Design review of the part shown in the three views and the two pictorial views. Dimensions are in mm from the part's minimum x, y and z. A direction names the side the tool comes from. Give positions to 0.01 mm unless a question says otherwise; leave off trailing zeros. Write each loop counter-clockwise with the first axis right and the second up, starting at its lowest first coordinate (ties: lowest second). Pieces come first, ordered by that corner, then holes. Notation, with made-up numbers: M 68,-32 L 90,-32 A17 ccw 90,-10 Z; hole C -17,67 d2. An arc over 180 degrees is marked long. Write item = value, one per line.
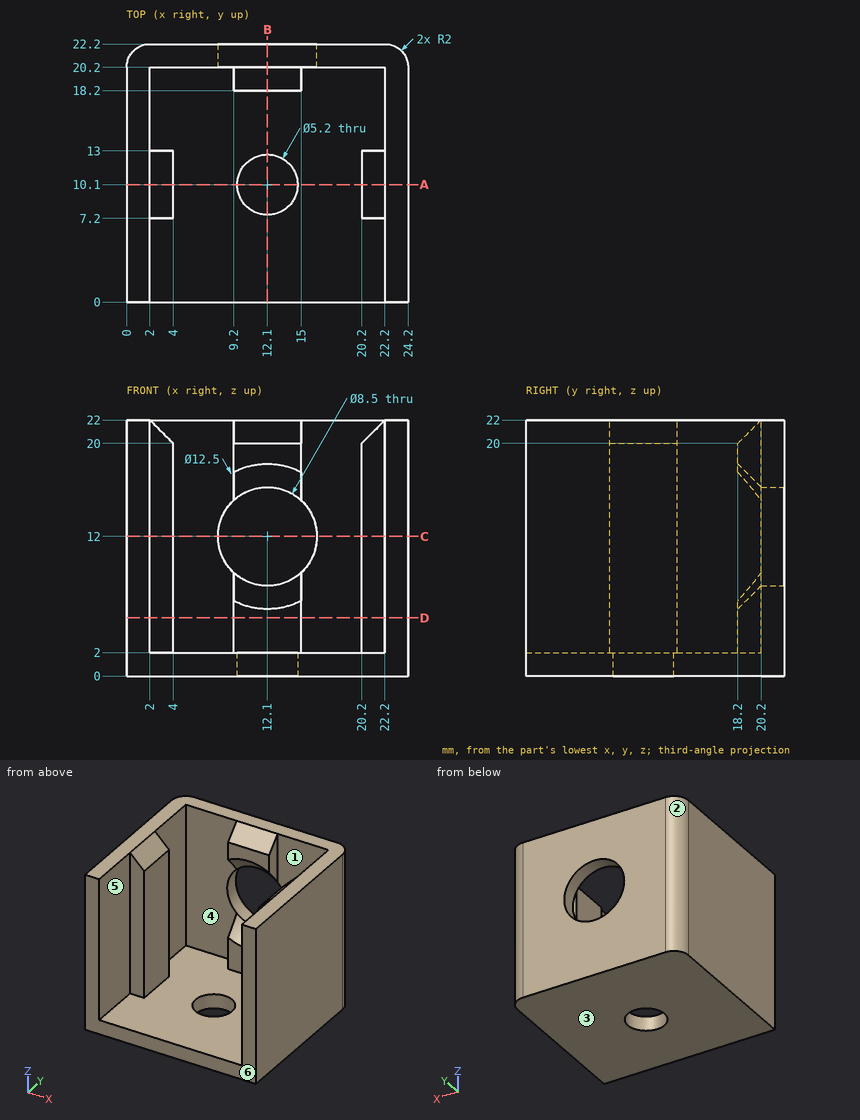
1. We need section D-D, the plane z = 5. Write out the cut boundary in (x, y), then the cut area to 3 significant figures.
Responses:
outline = M 0,0 L 2,0 L 2,7.2 L 4,7.2 L 4,13 L 2,13 L 2,20.2 L 9.2,20.2 L 9.2,18.2 L 15,18.2 L 15,20.2 L 22.2,20.2 L 22.2,13 L 20.2,13 L 20.2,7.2 L 22.2,7.2 L 22.2,0 L 24.2,0 L 24.2,20.2 A2 ccw 22.2,22.2 L 2,22.2 A2 ccw 0,20.2 Z
area = 162 mm2
2. Machinability: for the marked faces 4, 5 and 6, which of the approach directions +Z, -Z, +X, -X, +Y, -Y give a long, thin tool a straight path to every point of the face, cutting with its end or side? Answer none if there is none.
Responses:
face_4 = +Z
face_5 = +Z, -Y
face_6 = +Z, -Z, +X, -X, -Y
3. We need section C-C, the plane z = 12. Write out the cut boundary in (x, y), then the cut area to 3 significant figures.
Responses:
outline = M 0,0 L 2,0 L 2,7.2 L 4,7.2 L 4,13 L 2,13 L 2,20.2 L 7.85,20.2 L 7.85,22.2 L 2,22.2 A2 ccw 0,20.2 Z; M 16.35,20.2 L 22.2,20.2 L 22.2,13 L 20.2,13 L 20.2,7.2 L 22.2,7.2 L 22.2,0 L 24.2,0 L 24.2,20.2 A2 ccw 22.2,22.2 L 16.35,22.2 Z
area = 134 mm2
4. For line 1 along Y through (x, z) = (12.1, 0.7); line 2 along X through (y, z) = (19.75, 18.75); line 3 along Y through (x, z) = (22, 4.25), list the stretches that pass through material, from the lowest coordinate up. Write a range as from..to.
Responses:
line_1 = 0..7.5, 12.7..22.2
line_2 = 0..2, 9.2..15, 22.2..24.2
line_3 = 7.2..13, 20.2..22.2
5. Insertion check: P1, Ø0.7, axis at x = 12.5, z = 18.5, coming from the -Y side; P2, Ø2, axis at x = 6, z = 13.5, coming from the -Y side. Each pin has a flat end and moves straight along its axis. Give the tip position at first contact, or say it passes through.
Responses:
P1 = 18.2
P2 = 20.2
6. The part is to be moulded in two halves that separate along Y. For the marked faces 1, 2 and 3, say which applies: +Y half, -Y half, draft (parallel to the pull), parting line (faces both ways), or undercut.
Responses:
face_1 = undercut
face_2 = +Y half
face_3 = draft
7. We need section B-B, the plane x = 12.1. Write out the cut boundary in (y, z).
Responses:
outline = M 0,0 L 7.5,0 L 7.5,2 L 0,2 Z; M 12.7,0 L 22.2,0 L 22.2,7.75 L 20.2,7.75 L 18.2,5.75 L 18.2,2 L 12.7,2 Z; M 18.2,18.25 L 20.2,16.25 L 22.2,16.25 L 22.2,22 L 20.2,22 L 18.2,20 Z
8. We need section A-A, the plane y = 10.1. Write out the cut boundary in (x, z).
Responses:
outline = M 0,0 L 9.5,0 L 9.5,2 L 4,2 L 4,20 L 2,22 L 0,22 Z; M 14.7,0 L 24.2,0 L 24.2,22 L 22.2,22 L 20.2,20 L 20.2,2 L 14.7,2 Z
